Could you check a few things on this model? Use its own coordinates, in mm. A direction names the side the tool comes from. Give positions to 0.01 mm unless a question says otherwise; leave off trailing zeros. Order: outer loops, then holes, each group sorted by start corner. A loop starts at its lowest first (then second) coordinate and runs counter-clockwise, first axis right, second up. Notation, with made-up numbers: M 16.5,-5.5 L 64.5,-5.5 A26 ccw 64.5,26.5 Z; hole C -15.75,76.25 d11. An arc over 180 degrees is marked long. Return JSON: item names as keys, results as strings. Group by question number.
```python
from build123d import *

# Parameters (mm, degrees)
SKETCH_3_R      = 0.2
EXTRUDE_1_DEPTH = 10
SKETCH_4_R      = 0.2
EXTRUDE_2_DEPTH = 3


with BuildPart() as part:
    # 草图2 → 旋转1 (revolve)
    with BuildSketch(Plane(origin=(0, 0, 0), x_dir=(1, 0, 0), z_dir=(0, 1, 0))):
        with BuildLine():
            Line((2.36, -6.04), (2.36, -1))
            Line((2.36, -1), (2.7, -1))
            Line((2.7, -1), (2.7, 0))
            Line((2.7, 0), (0, 0))
            Line((0, 0), (0, -8.4))
            ThreePointArc((0, -8.4), (1.668772004, -7.708772004), (2.36, -6.04))
        make_face()
    revolve(axis=Axis((0, 0, 0), (0, 0, 1)))

    # 草图3 → 凸台-拉伸1 (add)
    with BuildSketch(Plane(origin=(0, 0, 0), x_dir=(-1, 0, 0), z_dir=(0, 0, -1))):
        with Locations((1.3, 0)):
            Circle(SKETCH_3_R)
        with Locations((-1.3, 0)):
            Circle(SKETCH_3_R)
    extrude(amount=EXTRUDE_1_DEPTH)

    # 草图4 → 凸台-拉伸2 (add)
    with BuildSketch(Plane(origin=(0, 0, -10), x_dir=(-1, 0, 0), z_dir=(0, 0, -1))):
        with Locations((1.3, 0)):
            Circle(SKETCH_4_R)
    extrude(amount=EXTRUDE_2_DEPTH)


solid = part.part
```
1. Imagine slicing it at D-D, the plane z = 0.5. Please give me the cut outline in (x, y), plus the area to 3 significant figures.
2. I need wall thicknesses on L1, parallel to Z at x = 0.4, y = 2.45; L2, parallel to Z at x = -1.7, y = 1.05; L3, parallel to Y at x = 1.55, z = 1.25. Which ranges of each line are inside material? Lowest first, please. Write a range as from..to.
3. Which directions (+Z, -Z, +X, -X, +Y, -Y) give clear straight access to the entire face, cutting with the end or side of a thin tool? Please do faces 1 (the cylindrical face through (-0.585, -2.636, 0.493)), 2 (the cylindrical face through (-1.9, -1.4, 3.5)).
4. Imagine slicing it at A-A, the plane y = 0. Please give me the cut outline in (x, z).
5. For pin 1 (1.5 mm diameter, centred on y = -1.5, z = 1.5, fed in from +X); pin 2 (1.5 mm diameter, centred on x = -1.5, y = 2, fed in from +Z); pin 3 (1.5 mm diameter, centred on x = 1, z = -9, fed in from -Y), each with a flat end and sliding along its axis, tell me the tip position at first contact or that it passes through.
6. Imagine slicing it at B-B, the plane z = -4.75. Please give me the cut outline in (x, y).
7. Imagine slicing it at C-C, the plane x = 1.3. Please give me the cut outline in (y, z).
Values:
{
 "1": {"outline": "C 0,0 d5.4", "area": "22.9 mm²"},
 "2": {"L1": "z = 0..1", "L2": "z = 0..7.3", "L3": "y = -1.78..1.78"},
 "3": {"face 1": "+Z, -Z", "face 2": "+Z"},
 "4": {"outline": "M -2.7,0 L -1.5,0 L -1.5,-13 L -1.1,-13 L -1.1,0 L 1.1,0 L 1.1,-10 L 1.5,-10 L 1.5,0 L 2.7,0 L 2.7,1 L 2.36,1 L 2.36,6.04 A2.36 ccw -2.36,6.04 L -2.36,1 L -2.7,1 Z"},
 "5": {"pin 1": "stops at x = 2.53", "pin 2": "stops at z = 7.62", "pin 3": "stops at y = -0.2"},
 "6": {"outline": "C -1.3,0 d0.4; C 1.3,0 d0.4"},
 "7": {"outline": "M -2.37,0 L -0.2,0 L -0.2,-10 L 0.2,-10 L 0.2,0 L 2.37,0 L 2.37,1 L 1.97,1 L 1.97,6.04 A1.97 ccw -1.97,6.04 L -1.97,1 L -2.37,1 Z"}
}
